Source: CAD feature listing. Evaluate the final solid. Frame: model axes, mm. Coordinates: 2 decimals unless noted, no trailing zeros. Order: outer loops, then holes, each group sorted by start corner. A loop starts at its lowest first (then second) coordinate and runs counter-clockwise, first axis right, second up.
Autodesk Inventor part; units mm, degrees
ref_plane "YZ Plane" through (0, 0, 0) normal (1, 0, 0) x (0, 1, 0)
ref_plane "XZ Plane" through (0, 0, 0) normal (0, 1, 0) x (-1, 0, 0)
ref_plane "XY Plane" through (0, 0, 0) normal (0, 0, 1) x (1, 0, 0)
sketch "Sketch1" plane through (0, 0, 0) normal (0, 1, 0) x (-1, 0, 0)
  circle A0 centre (0, 0) radius 150
  dimension "d0" = 300
extrude "Extrusion1" add sketch "Sketch1" along normal blind 2
sketch "Sketch2" plane through (0, 2, 0) normal (0, 1, 0) x (1, 0, 0)
  circle A0 centre (62.132, 62.132) radius 50
  circle A1 centre (0, 0) radius 150 construction
  line L0 (0, 150) -> (0, -150) construction
  line L1 (150, 0) -> (-150, 0) construction
  line L2 (62.132, 62.132) -> (0, 62.132) construction
  line L3 (62.132, 62.132) -> (62.132, 0) construction
  line L4 (62.132, 62.132) -> (106.066, 106.066) construction
  dimension "d3" = 100
  dimension "d26" = 62.132
extrude "Extrusion2" cut sketch "Sketch2" against normal through all
pattern_circular "Circular Pattern1" count 4 over 360 about axis through (0, -10, 0) along (0, 1, 0) of "Extrusion2"
sketch "Sketch3" plane through (0, 2, 0) normal (0, 1, 0) x (1, 0, 0)
  circle A0 centre (0, 0) radius 5
  dimension "d9" = 10
extrude "Extrusion3" cut sketch "Sketch3" against normal through all
sketch "Sketch5" plane through (0, 2, 0) normal (0, 1, 0) x (1, 0, 0)
  circle A0 centre (0, 0) radius 5 construction
  line L0 (0, 0) -> (-150, 0) construction
  arc A1 (-150, 0) -> (-150, 0) centre (0, 0) ccw construction
  line L1 (-60, -1) -> (-60, 1)
  line L2 (-60, 1) -> (-90, 1)
  line L3 (-90, 1) -> (-90, -1)
  line L4 (-90, -1) -> (-60, -1)
  line L5 (-60, 0) -> (-90, 0) construction
  point P0 (-75, 0)
  dimension "d19" = 2
  dimension "d20" = 30
extrude "Extrusion5" cut sketch "Sketch5" against normal through all
pattern_circular "Circular Pattern3" count 4 over 360 about axis through (0, -10, 0) along (0, 1, 0) of "Extrusion5"
properties part number "Plate" material "Aluminum 6061"
1. Section query D-D on x = 25. Return loops of the section in (y, z), plus the area to 3 significant figures.
Findings:
outline: (0, -147.9) - (2, -147.9) - (2, -95.62) - (0, -95.62) - close; (0, -28.65) - (2, -28.65) - (2, 28.65) - (0, 28.65) - close; (0, 95.62) - (2, 95.62) - (2, 147.9) - (0, 147.9) - close
area: 324 mm2
2. Pin query (flat end, axial travel): P1, Ø0.6, axis at y = 1, z = 79, coming from the +X side; P2, Ø1, axis at x = -91, y = 1.5, coming from the -Z side; P3, Ø1, axis at y = 1.5, z = -68.5, coming from the +X side. Return the tip coordinate at first contact, or that it passes through.
Findings:
P1: stops at x = 127.7
P2: stops at z = -119.62
P3: stops at x = 133.7
3. Section query A-A on x = -42. Return loops of the section in (y, z).
Findings:
outline: (0, -144) - (2, -144) - (2, -107.9) - (0, -107.9) - close; (0, -16.36) - (2, -16.36) - (2, 16.36) - (0, 16.36) - close; (0, 107.9) - (2, 107.9) - (2, 144) - (0, 144) - close
4. Draft query along Z for faces 1 (the face through (-31, 2, 2)), 2 (the face through (19.527, 0.986, -148.724)), 3 (the face through (42.98, 1.01, 108.32)). Return one class per face: released by +Z, released by -Z, zero draft, split by the parting line, or undercut.
Findings:
face 1: zero draft
face 2: split by the parting line
face 3: undercut
5. Ray query, line 1 (X direction, y = 1.5, z = 30); line 2 (Z direction, x = -70.5, y = 0.4); line 3 (X direction, y = 0.8, z = -62.5). Return the intervals inside material, ascending.
Findings:
line 1: x = -146.97 to -100.44, -23.82 to 23.82, 100.44 to 146.97
line 2: z = -132.4 to -111.43, -12.84 to -1, 1 to 12.84, 111.43 to 132.4
line 3: x = -136.36 to -112.13, -12.13 to -1, 1 to 12.13, 112.13 to 136.36
6. Section query B-B on z = -79. Return loops of the section in (x, y), plus the area to 3 significant figures.
Findings:
outline: (-127.51, 0) - (-109.2, 0) - (-109.2, 2) - (-127.51, 2) - close; (-15.06, 0) - (-1, 0) - (-1, 2) - (-15.06, 2) - close; (1, 0) - (15.06, 0) - (15.06, 2) - (1, 2) - close; (109.2, 0) - (127.51, 0) - (127.51, 2) - (109.2, 2) - close
area: 129 mm2
7. Section query C-C on y = 0.95. Count the separate pieces of the cut face and the enclosed holes in it, plus the area to 3 significant figures.
Findings:
separate pieces: 1
enclosed holes: 9
area: 39,000 mm2
